Part model, mm, in its own coordinate system. A direction names the side the tool comes from. Give positions to 0.01 mm unless a question says otherwise; leave off trailing zeros. Write each loop counter-clockwise with the first axis right and the second up, starting at its lowest first coordinate (ties: lowest second). Pieces come first, ordered by that corner, then holes. Notation, with made-up numbers: (16.5, 67) - (31.5, 67) arc R19 ccw to (31.5, 104) - close; hole circle Ø8 at (-27.75, -25.5). An arc over 180 degrees is marked (long way). Answer in a Markdown table with one row per item. Add a question column.
1. Band-saw the part on C-C on y = -50. Write the cut outline in (x, z), plus the area to 3 significant figures.
2. Probe line 1 along Z through (x, y) = (-92.5, 0); line 2 along Y through (x, z) = (0, -0.6); line 3 along X through (y, z) = (-9.5, 6.5). List the from-to ranges inside material, lowest first.
3. Pull direction X, two halves, no side cores. Call faces 1 (the flat face through (-79.5, 0, 41)), 2 (the flat face through (87, 0, 10)), 3 (the flat face through (94.5, 0, 41)): released by +X, released by -X, zero draft, split by the parting line, or undercut.
4. Which spindle directions (+Z, -Z, +X, -X, +Y, -Y) get a long thin tool onto all of the face, cutting with end or side? Do faces 4 (the cylindrical face through (82.95, 4.21, 71.85)), 5 (the flat face through (87, -20, 31)), 6 (the flat face through (87, -11, 25)). Say none if no direction does.
5. Drop flat-ended pins along their axis: pin 1 Ø6 at (x, y) = (-52, 48) entering from +Z; pin 2 Ø25 at (y, z) = (0, 58.5) entering from +X; pin 3 Ø20 at (y, z) = (5, 37.5) entering from -X. Give the stop position or say it passes through.
6. Band-saw the part on A-A on z = 26.5. Write the cut outline in (x, y).
7. Band-saw the part on B-B on z = 7.5. Write the cut outline in (x, y), plus the area to 3 significant figures.
8. Band-saw the part on D-D on x = 38. Write the cut outline in (y, z), plus the area to 3 significant figures.
```python
from build123d import *

# Parameters (mm, degrees)
SKETCH1_R           = 97.5
SKETCH1_R_2         = 16
BOSS_EXTRUDE1_DEPTH = 2.5
SKETCH2_R           = 5
CUT_EXTRUDE1_DEPTH  = 138.976447265
CIRPATTERN1_COUNT   = 4
CIRPATTERN1_ANGLE   = 180
SKETCH4_R           = 97.5
SKETCH4_R_2         = 94.5
BOSS_EXTRUDE2_DEPTH = 2
BOSS_EXTRUDE3_DEPTH = 7.5
SKETCH6_R           = 14
CUT_EXTRUDE2_DEPTH  = 7
CUT_EXTRUDE3_REACH  = 231.2
CUT_EXTRUDE4_REACH  = 159.444
SKETCH8_R           = 14
SKETCH9_R           = 14
CUT_EXTRUDE5_DEPTH  = 158.44364071


with BuildPart() as part:
    # Sketch1 → Boss-Extrude1 (new, symmetric)
    with BuildSketch(Plane.XY):
        Circle(SKETCH1_R)
        with Locations((38, 0)):
            Circle(SKETCH1_R_2, mode=Mode.SUBTRACT)
    extrude(amount=BOSS_EXTRUDE1_DEPTH, both=True)

    # Sketch2 → Cut-Extrude1 (cut, through all)
    with BuildSketch(Plane.XY.offset(2.5)):
        with Locations((0, 30)):
            Circle(SKETCH2_R)
    cut_extrude1 = extrude(amount=-CUT_EXTRUDE1_DEPTH, mode=Mode.SUBTRACT)

    # CirPattern1: Cut-Extrude1 ×4 about axis
    cirpattern1_axis = Axis((0, 0, 0), (0, 0, 1))
    for i in range(1, CIRPATTERN1_COUNT):
        add(cut_extrude1.rotate(cirpattern1_axis, i * CIRPATTERN1_ANGLE / (CIRPATTERN1_COUNT - 1)), mode=Mode.SUBTRACT)

    # Sketch4 → Boss-Extrude2 (add)
    with BuildSketch(Plane(origin=(0, 0, -2.5), x_dir=(-1, 0, 0), z_dir=(0, 0, -1))):
        Circle(SKETCH4_R)
        Circle(SKETCH4_R_2, mode=Mode.SUBTRACT)
    extrude(amount=BOSS_EXTRUDE2_DEPTH)

    # Sketch5 → Boss-Extrude3 (add, symmetric)
    with BuildSketch(Plane(origin=(87, 0, 0), x_dir=(0, 0, -1), z_dir=(1, 0, 0))):
        with BuildLine():
            Line((-2.5, 20), (-58.5, 20))
            ThreePointArc((-58.5, 20), (-44.357864376, 14.142135624), (-38.5, 0))
            ThreePointArc((-38.5, 0), (-44.357864376, -14.142135624), (-58.5, -20))
            Line((-58.5, -20), (-2.5, -20))
            Line((-2.5, -20), (-2.5, 20))
        make_face()
        with BuildLine():
            ThreePointArc((-38.5, 0), (-44.357864376, 14.142135624), (-58.5, 20))
            Line((-58.5, 20), (-58.5, 8.5))
            ThreePointArc((-58.5, 8.5), (-52.48959236, 6.01040764), (-50, 0))
            ThreePointArc((-50, 0), (-52.48959236, -6.01040764), (-58.5, -8.5))
            Line((-58.5, -8.5), (-58.5, -20))
            ThreePointArc((-58.5, -20), (-44.357864376, -14.142135624), (-38.5, 0))
        make_face()
        with BuildLine():
            Line((-58.5, 8.5), (-58.5, 20))
            ThreePointArc((-58.5, 20), (-78.5, 0), (-58.5, -20))
            Line((-58.5, -20), (-58.5, -8.5))
            ThreePointArc((-58.5, -8.5), (-67, 0), (-58.5, 8.5))
        make_face()
        with BuildLine():
            ThreePointArc((-38.5, 0), (-44.357864376, 14.142135624), (-58.5, 20))
            Line((-58.5, 20), (-58.5, 8.5))
            ThreePointArc((-58.5, 8.5), (-52.48959236, 6.01040764), (-50, 0))
            ThreePointArc((-50, 0), (-52.48959236, -6.01040764), (-58.5, -8.5))
            Line((-58.5, -8.5), (-58.5, -20))
            ThreePointArc((-58.5, -20), (-44.357864376, -14.142135624), (-38.5, 0))
        make_face()
        with BuildLine():
            Line((-58.5, 8.5), (-58.5, 20))
            ThreePointArc((-58.5, 20), (-78.5, 0), (-58.5, -20))
            Line((-58.5, -20), (-58.5, -8.5))
            ThreePointArc((-58.5, -8.5), (-67, 0), (-58.5, 8.5))
        make_face()
    boss_extrude3 = extrude(amount=BOSS_EXTRUDE3_DEPTH, both=True)

    # Sketch6 → Cut-Extrude2 (cut)
    with BuildSketch(Plane.ZY.offset(-79.5)):
        with Locations((58.5, 0)):
            Circle(SKETCH6_R)
    cut_extrude2 = extrude(amount=-CUT_EXTRUDE2_DEPTH, mode=Mode.SUBTRACT)

    # Sketch7 → Cut-Extrude3 (cut, up to next)
    with BuildSketch(Plane(origin=(94.5, 0, 0), x_dir=(0, 0, -1), z_dir=(1, 0, 0)), mode=Mode.PRIVATE) as cut_extrude3_sk1:
        with BuildLine():
            Line((-13, 11), (-37, 11))
            ThreePointArc((-37, 11), (-39.121320344, 10.121320344), (-40, 8))
            Line((-40, 8), (-40, -8))
            ThreePointArc((-40, -8), (-39.121320344, -10.121320344), (-37, -11))
            Line((-37, -11), (-13, -11))
            ThreePointArc((-13, -11), (-10.878679656, -10.121320344), (-10, -8))
            Line((-10, -8), (-10, 8))
            ThreePointArc((-10, 8), (-10.878679656, 10.121320344), (-13, 11))
        make_face()
    cut_extrude3_tool1 = extrude(cut_extrude3_sk1.sketch, amount=-CUT_EXTRUDE3_REACH, mode=Mode.PRIVATE) & part.part
    cut_extrude3 = cut_extrude3_tool1.solids().sort_by_distance((94.5, 0, 25))[0]
    add(cut_extrude3, mode=Mode.SUBTRACT)

    # Mirror1: Boss-Extrude3, Cut-Extrude2, Cut-Extrude3 across plane
    add(boss_extrude3.mirror(Plane(origin=(0, 0, 0), x_dir=(0, 0, 1), z_dir=(1, 0, 0))))
    add(cut_extrude2.mirror(Plane(origin=(0, 0, 0), x_dir=(0, 0, 1), z_dir=(1, 0, 0))), mode=Mode.SUBTRACT)
    add(cut_extrude3.mirror(Plane(origin=(0, 0, 0), x_dir=(0, 0, 1), z_dir=(1, 0, 0))), mode=Mode.SUBTRACT)

    # Sketch8 → Cut-Extrude4 (cut, up to next)
    with BuildSketch(Plane.XY.offset(2.5), mode=Mode.PRIVATE) as cut_extrude4_sk1:
        with Locations((-41, -50)):
            Circle(SKETCH8_R)
    cut_extrude4_tool1 = extrude(cut_extrude4_sk1.sketch, amount=-CUT_EXTRUDE4_REACH, mode=Mode.PRIVATE) & part.part
    add(cut_extrude4_tool1.solids().sort_by_distance((-41, -50, 2.5))[0], mode=Mode.SUBTRACT)

    # Sketch9 → Cut-Extrude5 (cut, through all)
    with BuildSketch(Plane.XY.offset(2.5)):
        with Locations((-23.540161495, 58)):
            Circle(SKETCH9_R)
    extrude(amount=-CUT_EXTRUDE5_DEPTH, mode=Mode.SUBTRACT)


solid = part.part
```
Values:
| question | item | result |
|---|---|---|
| 1 | outline | (-83.7, -4.5) - (-80.19, -4.5) - (-80.19, -2.5) - (-55, -2.5) - (-55, 2.5) - (-83.7, 2.5) - close; (-27, -2.5) - (80.19, -2.5) - (80.19, -4.5) - (83.7, -4.5) - (83.7, 2.5) - (-27, 2.5) - close |
| 1 | area | 711 mm² |
| 2 | line 1 | z = -2.5 to 10, 40 to 50, 67 to 78.5 |
| 2 | line 2 | y = -97.5 to -35, -25 to 25, 35 to 97.5 |
| 2 | line 3 | x = -94.5 to -79.5, 79.5 to 94.5 |
| 3 | face 1 | undercut |
| 3 | face 2 | zero draft |
| 3 | face 3 | released by +X |
| 4 | face 4 | none |
| 4 | face 5 | +Z, +X, -X, -Y |
| 4 | face 6 | +X, -X |
| 5 | pin 1 | stops at z = 2.5 |
| 5 | pin 2 | stops at x = 94.5 |
| 5 | pin 3 | stops at x = -94.5 |
| 6 | outline | (-94.5, -20) - (-79.5, -20) - (-79.5, -11) - (-94.5, -11) - close; (-94.5, 11) - (-79.5, 11) - (-79.5, 20) - (-94.5, 20) - close; (79.5, -20) - (94.5, -20) - (94.5, -11) - (79.5, -11) - close; (79.5, 11) - (94.5, 11) - (94.5, 20) - (79.5, 20) - close |
| 7 | outline | (-94.5, -20) - (-79.5, -20) - (-79.5, 20) - (-94.5, 20) - close; (79.5, -20) - (94.5, -20) - (94.5, 20) - (79.5, 20) - close |
| 7 | area | 1,200 mm² |
| 8 | outline | (-89.79, -4.5) - (-86.52, -4.5) - (-86.52, -2.5) - (-16, -2.5) - (-16, 2.5) - (-89.79, 2.5) - close; (16, -2.5) - (86.52, -2.5) - (86.52, -4.5) - (89.79, -4.5) - (89.79, 2.5) - (16, 2.5) - close |
| 8 | area | 751 mm² |
